Here's how the part is built. I have some questions about the finished solid (model axes, mm). A direction names the side the tool comes from. Round coordinates to 2 decimals unless told otherwise and drop trailing zeros. Loops run counter-clockwise (first coordinate to the right, second up) from the corner with the lowest first, then second, coordinate; pieces in that order, holes last. Notation, with made-up numbers: M 8.5,48 L 46.5,48 A19 ccw 46.5,62 Z; hole C 55,12.5 d6. An arc over 180 degrees is marked long. Answer as a JSON object with one key per item and string values.
from build123d import *

# Parameters (mm, degrees)
F0_W     = 30
F0_H     = 30
F1_DEPTH = 2
F2_DEPTH = 4
F3_R     = 2
F4_SIZE  = 0.5
F5_R     = 1
F6_R     = 1


with BuildPart() as f1:
    # F0 (on Top) → F1 (new body)
    with BuildSketch(Plane.XY):
        Rectangle(F0_W, F0_H)
        Polygon((-13.4, 13.4), (13.4, 13.4), (13.4, 4.1756560095), (13.4, -13.4), (-13.4, -13.4), (-13.4, 4.1756560095), align=None, mode=Mode.SUBTRACT)
        Polygon((13.4, 4.1756560095), (13.4, 13.4), (-13.4, 13.4), (-13.4, 4.1756560095), (-10.9, 4.1756560095), (-10.9, -10.9), (10.9, -10.9), (10.9, 4.1756560095), align=None)
        Polygon((13.4, -13.4), (13.4, 4.1756560095), (10.9, 4.1756560095), (10.9, -10.9), (-10.9, -10.9), (-10.9, 4.1756560095), (-13.4, 4.1756560095), (-13.4, -13.4), align=None)
    extrude(amount=F1_DEPTH)

    # F0 (on Top) → F2 (join)
    with BuildSketch(Plane.XY):
        Polygon((13.4, -13.4), (13.4, 4.1756560095), (10.9, 4.1756560095), (10.9, -10.9), (-10.9, -10.9), (-10.9, 4.1756560095), (-13.4, 4.1756560095), (-13.4, -13.4), align=None)
    extrude(amount=F2_DEPTH)

    # F3
    f3_edges = [f1.edges().sort_by_distance(p)[0] for p in [
        (-15, -15, 1),
        (-15, 15, 1),
        (15, 15, 1),
        (15, -15, 1),
    ]]
    fillet(f3_edges, radius=F3_R)

    # F4
    f4_edges = [f1.edges().sort_by_distance(p)[0] for p in [
        (13.4, -4.612172, 4),
        (0, -13.4, 4),
        (-13.4, -4.612172, 4),
    ]]
    chamfer(f4_edges, length=F4_SIZE)

    # F5
    f5_edges = [f1.edges().sort_by_distance(p)[0] for p in [
        (0, 15, 0),
    ]]
    fillet(f5_edges, radius=F5_R)

    # F6
    f6_edges = [f1.edges().sort_by_distance(p)[0] for p in [
        (13.4, -13.4, 2.75),
        (-13.4, -13.4, 2.75),
    ]]
    fillet(f6_edges, radius=F6_R)


solid = f1.part
Item 1: I want a section at C-C, the plane y = -1.75. Please give me the cut outline in (x, z), then the cut area to 3 significant figures.
Resolved:
{"outline": "M -15,1 A1 ccw -14,0 L 14,0 A1 ccw 15,1 L 15,2 L 13.4,2 L 13.4,3.5 L 12.9,4 L 10.9,4 L 10.9,2 L -10.9,2 L -10.9,4 L -12.9,4 L -13.4,3.5 L -13.4,2 L -15,2 Z", "area": "69.3 mm²"}
Item 2: I want a section at D-D, the plane x = 11.5. Please give me the cut outline in (y, z), then the cut area to 3 significant figures.
Resolved:
{"outline": "M -15,1 A1 ccw -14,0 L 14,0 A1 ccw 15,1 L 15,2 L 4.18,2 L 4.18,4 L -12.9,4 L -13.4,3.5 L -13.4,2 L -15,2 Z", "area": "94.6 mm²"}
Item 3: I'm going to push flat-ended pins straight in: pin 1 Ø1 at (y, z) = (-6, 3) entering from +X; pin 2 Ø15 at (x, y) = (-2.5, 4) entering from +Z; pin 3 Ø0.6 at (x, z) = (11.5, 3) entering from +Y. Where does each tip first touch, or does it pass through?
Resolved:
{"pin 1": "x = 13.4", "pin 2": "z = 2", "pin 3": "y = 4.18"}
Item 4: I want a section at B-B, the plane z = 2.55. Please give me the cut outline in (x, y).
Resolved:
{"outline": "M -13.4,-12.4 A1 ccw -12.4,-13.4 L 12.4,-13.4 A1 ccw 13.4,-12.4 L 13.4,4.18 L 10.9,4.18 L 10.9,-10.9 L -10.9,-10.9 L -10.9,4.18 L -13.4,4.18 Z"}
Item 5: Please list where these lines run through material, in increasing order: probe 1 along X at (y, z) = (-0.5, 2.15); probe 2 along Z at (x, y) = (-1, 12.75); probe 3 along Y at (x, z) = (7.5, 2.7). Write a range as from..to.
Resolved:
{"probe 1": "-13.4..-10.9, 10.9..13.4", "probe 2": "0..2", "probe 3": "-13.4..-10.9"}
Item 6: On a 3-axis mill with a long thin cutter (end or side, diameter ignored), from which of +Z, -Z, +X, -X, +Y, -Y can I reach the whole of each face in a straight line? I mean faces 1 (the face through (13.099, -13.115, 2.71)), 2 (the face through (0, -13.4, 3)), 3 (the face through (12, 4.176, 3)), 4 (the face through (10.9, -3, 3)), 5 (the face through (13.4, -4, 3)). Say none if no direction works.
Resolved:
{"face 1": "+Z, +X, -Y", "face 2": "+Z, +X, -X, -Y", "face 3": "+Z, +X, -X, +Y", "face 4": "+Z, +Y", "face 5": "+Z, +X, +Y, -Y"}
Item 7: I want a section at A-A, the plane x = 5.25. Please give me the cut outline in (y, z).
Resolved:
{"outline": "M -15,1 A1 ccw -14,0 L 14,0 A1 ccw 15,1 L 15,2 L -10.9,2 L -10.9,4 L -12.9,4 L -13.4,3.5 L -13.4,2 L -15,2 Z"}
